Input: dimensioned drawing with shaded views. Units: mm. Origin: part minimum x, y, z. Round coordinates to 2 decimals unless told otherwise and drop trailing zeros. Loops run counter-clockwise (first coordinate to the right, second up) from the corner with the lowest first, then second, coordinate; pieces in that order, holes last. Notation, with made-up numbers: (13.5, 5.25) -> (46.5, 5.25) arc R19 cw to (46.5, 26.25) -> close; hole circle Ø9 at (75.5, 16). An arc over 180 degrees is marked (long way). Answer as a JSON object with one key per item and string values.
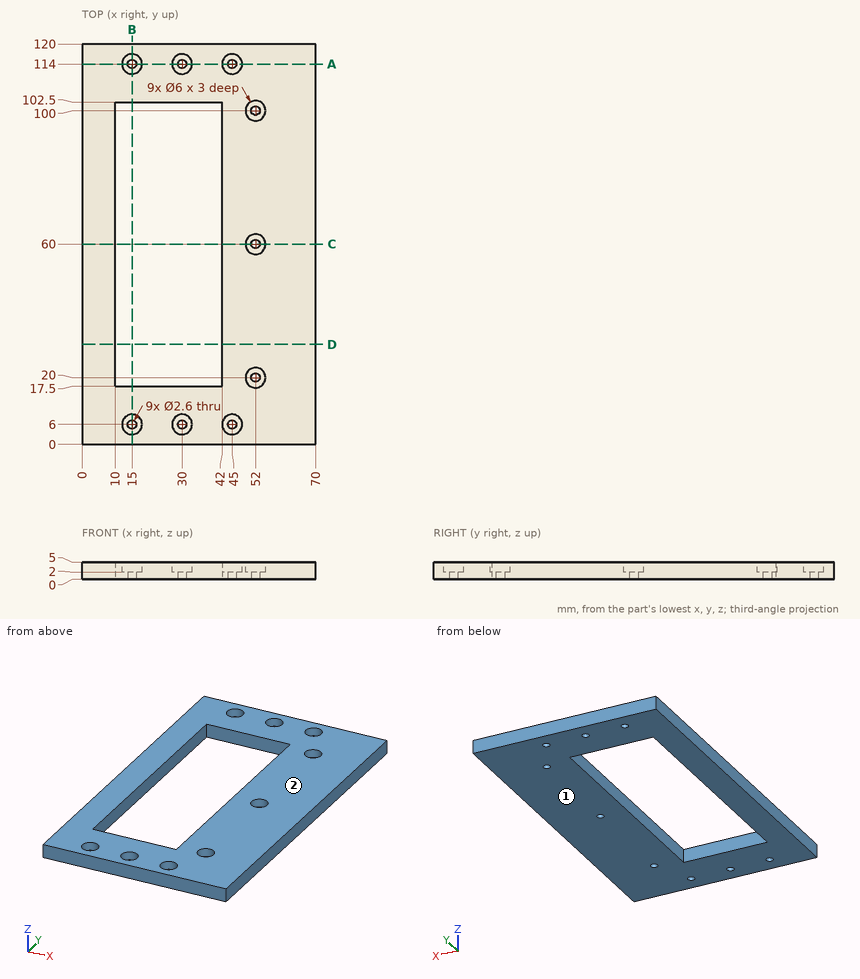
1) Section A-A, the plane y = 114. Output: boundary loops of the cut face in (x, z), plus the area to 3 significant figures.
Output:
{"outline": "(0, 0) -> (13.7, 0) -> (13.7, 2) -> (12, 2) -> (12, 5) -> (0, 5) -> close; (16.3, 0) -> (28.7, 0) -> (28.7, 2) -> (27, 2) -> (27, 5) -> (18, 5) -> (18, 2) -> (16.3, 2) -> close; (31.3, 0) -> (43.7, 0) -> (43.7, 2) -> (42, 2) -> (42, 5) -> (33, 5) -> (33, 2) -> (31.3, 2) -> close; (46.3, 0) -> (70, 0) -> (70, 5) -> (48, 5) -> (48, 2) -> (46.3, 2) -> close", "area": "280 mm^2"}
2) Section B-B, the plane x = 15. Output: boundary loops of the cut face in (y, z), plus the area to 3 significant figures.
Output:
{"outline": "(0, 0) -> (4.7, 0) -> (4.7, 2) -> (3, 2) -> (3, 5) -> (0, 5) -> close; (7.3, 0) -> (17.5, 0) -> (17.5, 5) -> (9, 5) -> (9, 2) -> (7.3, 2) -> close; (102.5, 0) -> (112.7, 0) -> (112.7, 2) -> (111, 2) -> (111, 5) -> (102.5, 5) -> close; (115.3, 0) -> (120, 0) -> (120, 5) -> (117, 5) -> (117, 2) -> (115.3, 2) -> close", "area": "129 mm^2"}
3) Contact query for a flat-ended pin moving along its axis: P1, Ø1.8, axis at x = 46, y = 114.5, coming from the +Z side. Output: stop coordinate, or through.
Output:
{"P1": "stops at z = 2"}
4) Ray query, probe 1 along X at (y, z) = (114, 1.3); probe 2 along Y at (x, z) = (15, 2.55); probe 3 along Y at (x, z) = (52, 0.4). Return the intervals inside material, ascending.
Output:
{"probe 1": "x = 0 to 13.7, 16.3 to 28.7, 31.3 to 43.7, 46.3 to 70", "probe 2": "y = 0 to 3, 9 to 17.5, 102.5 to 111, 117 to 120", "probe 3": "y = 0 to 18.7, 21.3 to 58.7, 61.3 to 98.7, 101.3 to 120"}
5) Section C-C, the plane y = 60. Output: boundary loops of the cut face in (x, z), plus the area to 3 significant figures.
Output:
{"outline": "(0, 0) -> (10, 0) -> (10, 5) -> (0, 5) -> close; (42, 0) -> (50.7, 0) -> (50.7, 2) -> (49, 2) -> (49, 5) -> (42, 5) -> close; (53.3, 0) -> (70, 0) -> (70, 5) -> (55, 5) -> (55, 2) -> (53.3, 2) -> close", "area": "167 mm^2"}
6) Draft query along Z for the marked faces 1 and 2. Return one class per face: +Z half, -Z half, draft (parallel to the pull), parting line (faces both ways), or undercut.
Output:
{"face 1": "-Z half", "face 2": "+Z half"}
7) Section D-D, the plane y = 30. Output: boundary loops of the cut face in (x, z), plus the area to 3 significant figures.
Output:
{"outline": "(0, 0) -> (10, 0) -> (10, 5) -> (0, 5) -> close; (42, 0) -> (70, 0) -> (70, 5) -> (42, 5) -> close", "area": "190 mm^2"}
